from build123d import *

# Parameters (mm, degrees)
SKETCH1_R           = 7
SKETCH1_R_2         = 5.25
BOSS_EXTRUDE1_DEPTH = 2.5
SKETCH2_R           = 7
BOSS_EXTRUDE2_DEPTH = 1
SKETCH3_R           = 7
SKETCH3_R_2         = 4.25
BOSS_EXTRUDE3_DEPTH = 2.5


with BuildPart() as part:
    # Sketch1 → Boss-Extrude1 (new body)
    with BuildSketch(Plane(origin=(0, 0, 0), x_dir=(1, 0, 0), z_dir=(0, 1, 0))):
        Circle(SKETCH1_R)
        Circle(SKETCH1_R_2, mode=Mode.SUBTRACT)
    extrude(amount=BOSS_EXTRUDE1_DEPTH)

    # Sketch2 → Boss-Extrude2 (add)
    with BuildSketch(Plane(origin=(0, 2.5, 0), x_dir=(1, 0, 0), z_dir=(0, 1, 0))):
        Circle(SKETCH2_R)
    extrude(amount=BOSS_EXTRUDE2_DEPTH)

    # Sketch3 → Boss-Extrude3 (add)
    with BuildSketch(Plane(origin=(0, 3.5, 0), x_dir=(1, 0, 0), z_dir=(0, 1, 0))):
        Circle(SKETCH3_R)
        Circle(SKETCH3_R_2, mode=Mode.SUBTRACT)
    extrude(amount=BOSS_EXTRUDE3_DEPTH)


solid = part.part
Input: part model. Units: mm. Frame: model coordinates. A direction names the side the tool comes from. Give positions to 0.01 mm unless a question says otherwise; leave off trailing zeros. Loops run counter-clockwise (first coordinate to the right, second up) from the corner with the lowest first, then second, coordinate; pieces in that order, holes last. Notation, with made-up numbers: (54.25, -17.5) -> (68.25, -17.5) arc R25 ccw to (68.25, 13.5) -> close; hole circle Ø3 at (-3, 20.25). An arc over 180 degrees is marked (long way). Answer as a JSON object with one key per item and string values. Group by question number.
Item 1: Pin query (flat end, axial travel): P1, Ø2, axis at x = -2, z = 2.5, coming from the +Y side; P2, Ø1.5, axis at y = 4, z = -4.5, coming from the +X side; P3, Ø7, axis at x = 0, z = 0, coming from the -Y side. Return the tip coordinate at first contact, or that it passes through.
Item 2: Cut plane A-A, the plane x = 0. Return the cut outline in (y, z), and give its area (3 significant figures).
Item 3: Cut plane C-C, the plane z = 0. Return the cut outline in (x, y).
Item 4: Reachability of faces 1 (the flat face through (3, 0, -5)), 2 (the cylindrical face through (2.285, 4.732, -3.584)), 3 (the flat face through (0, 2.5, 0)) from +Z, -Z, +X, -X, +Y, -Y: full face, straight path, thin tool, end or side. Return the list, or none.
Item 5: Pull-direction query (X, two-part tool) for faces 4 (the cylindrical face through (5, 1.2, -1.6)), 5 (the flat face through (0, 6, 5)), 6 (the cylindrical face through (6.466, 2.958, 2.681)); classes: released by +X, released by -X, zero draft, split by the parting line, or undercut.
Item 6: Cut plane D-D, the plane y = 2.8. Return the cut outline in (x, z), and give its area (3 significant figures).
Item 7: Line query: probe 1 along X at (y, z) = (1.5, 0); probe 2 along X at (y, z) = (4.2, 0). Output: solid intervals per line, ascending.
Item 8: Cut plane B-B, the plane y = 1.7. Return the cut outline in (x, z), and give its area (3 significant figures).
Checks:
{
 "1": {"P1": "stops at y = 3.5", "P2": "stops at x = 5.91", "P3": "stops at y = 2.5"},
 "2": {"outline": "(0, -7) -> (6, -7) -> (6, -4.25) -> (3.5, -4.25) -> (3.5, 4.25) -> (6, 4.25) -> (6, 7) -> (0, 7) -> (0, 5.25) -> (2.5, 5.25) -> (2.5, -5.25) -> (0, -5.25) -> close", "area": "36.5 mm²"},
 "3": {"outline": "(-7, 0) -> (-5.25, 0) -> (-5.25, 2.5) -> (5.25, 2.5) -> (5.25, 0) -> (7, 0) -> (7, 6) -> (4.25, 6) -> (4.25, 3.5) -> (-4.25, 3.5) -> (-4.25, 6) -> (-7, 6) -> close"},
 "4": {"face 1": "+Z, -Z, +X, -X, -Y", "face 2": "+Y", "face 3": "-Y"},
 "5": {"face 4": "undercut", "face 5": "zero draft", "face 6": "split by the parting line"},
 "6": {"outline": "circle Ø14 at (0, 0)", "area": "154 mm²"},
 "7": {"probe 1": "x = -7 to -5.25, 5.25 to 7", "probe 2": "x = -7 to -4.25, 4.25 to 7"},
 "8": {"outline": "circle Ø14 at (0, 0); hole circle Ø10.5 at (0, 0)", "area": "67.3 mm²"}
}
